Work out the finished part from the listing and answer in its coordinate system (mm). Face numbers are marked on the shaded views. Coordinates: 2 decimals unless noted, no trailing zeros. Write each loop counter-clockwise with the first axis right and the second up, starting at its lowest first coordinate (ties: lowest second). Pieces come first, ordered by that corner, then holes. Notation, with made-up numbers: (-30, 61) - (6, 61) arc R13 cw to (6, 67) - close; hole circle Ø10 at (4, 43.5). An arc over 180 degrees is marked (long way). One line per item, written item: value.
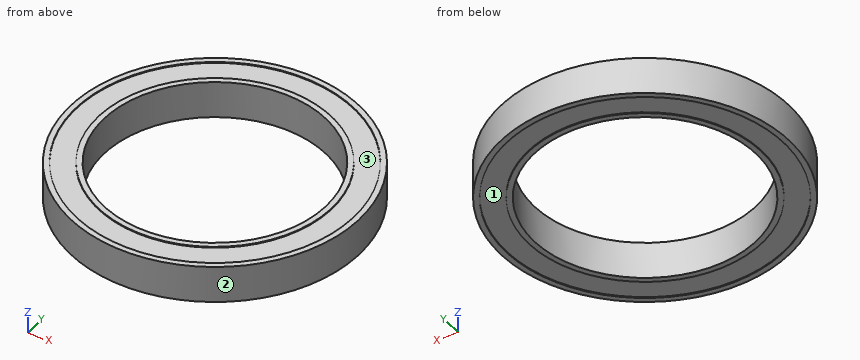
Autodesk Inventor part; units mm, degrees
ref_plane "YZ Plane" through (0, 0, 0) normal (1, 0, 0) x (0, 1, 0)
ref_plane "XZ Plane" through (0, 0, 0) normal (0, 1, 0) x (-1, 0, 0)
ref_plane "XY Plane" through (0, 0, 0) normal (0, 0, 1) x (1, 0, 0)
sketch "Sketch1" plane through (0, 0, 0) normal (0, 0, 1) x (1, 0, 0)
  circle A0 centre (0, 0) radius 30
  circle A1 centre (0, 0) radius 39
  circle A2 centre (0, 0) radius 37.5
  circle A3 centre (0, 0) radius 31.5
  dimension "d0" = 60
  dimension "d1" = 78
  dimension "d2" = 1.5
  dimension "d3" = 1.5
extrude "Extrusion1" add sketch "Sketch1" along normal mid plane 10
extrude "Extrusion2" add sketch "Sketch1" along normal mid plane 9.5 contours A2
properties part number "6812ZZ" material "Steel, Carbon"
Item 1: Given pin 1 (1 mm diameter, centred on y = -2, z = 0.5, fed in from +X); pin 2 (1 mm diameter, centred on y = 29.5, z = 3.5, fed in from +X); pin 3 (6 mm diameter, centred on x = 7.5, z = -1.5, fed in from -Y), each flat-ended and moving along its own axis, determine where each tip first touches the part or whether it passes through.
Evaluation:
pin 1: stops at x = 38.97
pin 2: stops at x = 26.08
pin 3: stops at y = -38.74
Item 2: Section D-D, the plane y = 34 is taken. Determine the outline of the cut face in (x, z).
Evaluation:
outline: (-19.1, -5) - (-15.82, -5) - (-15.82, -4.75) - (15.82, -4.75) - (15.82, -5) - (19.1, -5) - (19.1, 5) - (15.82, 5) - (15.82, 4.75) - (-15.82, 4.75) - (-15.82, 5) - (-19.1, 5) - close
Item 3: Section C-C, the plane z = -1.75 is taken. Determine the outline of the cut face in (x, y).
Evaluation:
outline: circle Ø78 at (0, 0); hole circle Ø60 at (0, 0)
Item 4: Section A-A, the plane y = 0 is taken. Determine the outline of the cut face in (x, z).
Evaluation:
outline: (-39, -5) - (-37.5, -5) - (-37.5, -4.75) - (-31.5, -4.75) - (-31.5, -5) - (-30, -5) - (-30, 5) - (-31.5, 5) - (-31.5, 4.75) - (-37.5, 4.75) - (-37.5, 5) - (-39, 5) - close; (30, -5) - (31.5, -5) - (31.5, -4.75) - (37.5, -4.75) - (37.5, -5) - (39, -5) - (39, 5) - (37.5, 5) - (37.5, 4.75) - (31.5, 4.75) - (31.5, 5) - (30, 5) - close
Item 5: Determine the mould class of the marked faces 1, 2 and 3 for opening direction Y: +Y half, -Y half, draft (parallel to the pull), parting line (faces both ways), or undercut.
Evaluation:
face 1: undercut
face 2: parting line
face 3: undercut
Item 6: Consider probe 1 along Y at (x, z) = (0, -4.85); probe 2 along Y at (x, z) = (19, 0.5); probe 3 along Z at (x, y) = (-8.5, 32). Determine where each line is inside the solid, lowest interval first.
Evaluation:
probe 1: y = -39 to -37.5, -31.5 to -30, 30 to 31.5, 37.5 to 39
probe 2: y = -34.06 to -23.22, 23.22 to 34.06
probe 3: z = -4.75 to 4.75
